Read the model definition and answer for the solid it produces. Units are mm, in the model's axes. Coordinates: 2 decimals unless noted, no trailing zeros. Write each loop counter-clockwise with the first axis right and the second up, starting at its lowest first coordinate (ties: lowest second). Pieces come first, ordered by that corner, then holes.
1) The part is cut by section D-D (x = -33). Determine the outline of the cut face in (y, z).
2) Each of these flat-tipped pins is pushed along its axis until it touches: pin 1 Ø3 at (x, y) = (-35.5, 1.5) entering from +Z; pin 2 Ø4 at (x, z) = (-39.5, 6) entering from -Y; pin 3 Ø2 at (y, z) = (6.5, 2.5) entering from +X; pin 4 Ø2 at (x, z) = (-27, 1) entering from +Y. Where does it stop, or does it pass through?
3) The part is cut by section C-C (z = 6.25). Determine the outline of the cut face in (x, y), then the cut area to 3 significant figures.
4) The part is cut by section B-B (z = 0.5). Determine the outline of the cut face in (x, y).
5) Determine the mould class of faces 1 (the face through (-28, -2.5, 3)), 2 (the face through (-11, 0, 0)), 3 (the face through (-28, 2.5, 3)), 4 (the face through (-6, 0, 2)) for opening direction Y: +Y half, -Y half, draft (parallel to the pull), parting line (faces both ways), or undercut.
6) The part is cut by section A-A (x = 0). Determine the outline of the cut face in (y, z), then the cut area to 3 significant figures.
7) Find the intervals of material crossed by line 1 (Y direction, x = 0, z = 3.05); line 2 (X direction, y = 0.75, z = 2.25); line 3 (Y direction, x = -14, z = 0.5), in increasing order.
from build123d import *

# Parameters (mm, degrees)
F0_R     = 6
F1_DEPTH = 4
F0_W     = 1.5
F0_H     = 5
F0_W_2   = 10.35
F0_W_3   = 4
F2_DEPTH = 7
F6_SIZE  = 2.99999


# Not quite as in the source:
# - a fillet or chamfer is up to 0.001 mm smaller than in the source, because OpenCascade refuses the exact size


with BuildPart() as f1:
    # F0 (on Top) → F1 (new body)
    with BuildSketch(Plane.XY):
        with BuildLine():
            ThreePointArc((-10.7121426428, -2.5), (1.258258902, -10.9277987049), (11, 0))
            ThreePointArc((11, 0), (1.258258902, 10.9277987049), (-10.7121426428, 2.5))
            ThreePointArc((-10.7121426428, 2.5), (-11, 0), (-10.7121426428, -2.5))
        make_face()
        Circle(F0_R, mode=Mode.SUBTRACT)
    extrude(amount=F1_DEPTH)

    # F0 (on Top) → F2 (join)
    with BuildSketch(Plane.XY):
        with BuildLine():
            ThreePointArc((-10.7121426428, -2.5), (-11, 0), (-10.7121426428, 2.5))
            Line((-10.7121426428, 2.5), (-15.0121426428, 2.5))
            Line((-15.0121426428, 2.5), (-15.0121426428, -2.5))
            Line((-15.0121426428, -2.5), (-10.7121426428, -2.5))
        make_face()
        with Locations((-15.7621426428, 0)):
            Rectangle(F0_W, F0_H)
        with Locations((-17.2621426428, 0)):
            Rectangle(F0_W, F0_H)
        with Locations((-33.5371426428, 0)):
            Rectangle(F0_W_2, F0_H)
        with Locations((-39.4621426428, 0)):
            Rectangle(F0_W, F0_H)
        with Locations((-40.9621426428, 0)):
            Rectangle(F0_W, F0_H)
        with Locations((-43.7121426428, 0)):
            Rectangle(F0_W_3, F0_H)
        with Locations((-23.1871426428, 0)):
            Rectangle(F0_W_2, F0_H)
    extrude(amount=F2_DEPTH)

    # F6 (size 3 in the source; OpenCascade refuses exactly that, so slightly less here)
    f6_edges = [f1.edges().sort_by_distance(p)[0] for p in [
        (-11, 0, 7),
    ]]
    chamfer(f6_edges, length=F6_SIZE)


with BuildPart() as f3:
    # F0 (on Top) → F3 (revolve)
    with BuildSketch(Plane.XY):
        with Locations((-15.7621426428, 0)):
            Rectangle(F0_W, F0_H)
    revolve(axis=Axis((-16.5121426428, 0, 0), (0, -1, 0)))


with BuildPart() as f4:
    # F0 (on Top) → F4 (revolve)
    with BuildSketch(Plane.XY):
        with Locations((-39.4621426428, 0)):
            Rectangle(F0_W, F0_H)
    revolve(axis=Axis((-40.2121426428, 0, 0), (0, -1, 0)))


with BuildPart() as f4_1:
    # F5: moved
    add(f4.part.moved(Location((0, 0, 3.5))))


with BuildPart() as f3_1:
    # F5: moved
    add(f3.part.moved(Location((0, 0, 3.5))))


with BuildPart() as f7:
    # F0 (on Top) → F7 (revolve)
    with BuildSketch(Plane.XY):
        with Locations((-23.1871426428, 0)):
            Rectangle(F0_W_2, F0_H)
    revolve(axis=Axis((-28.3621426428, 0, 0), (0, -1, 0)))


with BuildPart() as f7_1:
    # F8: moved
    add(f7.part.moved(Location((0, 0, 13.8))))


with BuildPart() as f1_1:
    add(f1.part)

    # F9: cut F4, F7, F3
    add(f4_1.part, mode=Mode.SUBTRACT)
    add(f7_1.part, mode=Mode.SUBTRACT)
    add(f3_1.part, mode=Mode.SUBTRACT)


solid = f1_1.part
Reported:
1. outline: (-2.5, 0) - (2.5, 0) - (2.5, 4.55) - (-2.5, 4.55) - close
2. pin 1: stops at z = 7
2. pin 2: stops at y = -2.5
2. pin 3: stops at x = 9.53
2. pin 4: stops at y = 2.5
3. outline: (-45.71, -2.5) - (-35.44, -2.5) - (-35.44, 2.5) - (-45.71, 2.5) - close; (-21.28, -2.5) - (-13.01, -2.5) arc R13.25 cw to (-13.01, 2.5) - (-21.28, 2.5) - close
3. area: 91.9 mm2
4. outline: (-45.71, -2.5) - (-10.71, -2.5) arc R11 ccw (long way) to (-10.71, 2.5) - (-45.71, 2.5) - close; hole circle Ø12 at (0, 0)
5. face 1: -Y half
5. face 2: draft
5. face 3: +Y half
5. face 4: undercut
6. outline: (-11, 0) - (-6, 0) - (-6, 4) - (-11, 4) - close; (6, 0) - (11, 0) - (11, 4) - (6, 4) - close
6. area: 40.0 mm2
7. line 1: y = -11 to -6, 6 to 11
7. line 2: x = -45.71 to -41.04, -39.38 to -17.34, -15.68 to -5.95, 5.95 to 10.97
7. line 3: y = -2.5 to 2.5
